Build history of the part. All positions in model axes, mm. Give positions to 0.01 mm unless a question says otherwise; leave off trailing zeros. Loops run counter-clockwise (first coordinate to the right, second up) from the corner with the lowest first, then second, coordinate; pieces in that order, holes last. Notation, with made-up numbers: (75.5, 34.25) -> (99.5, 34.25) arc R30 cw to (99.5, 56.25) -> close; hole circle Ø7 at (-21.75, 68). An arc over 180 degrees is marked (long way). Answer as a JSON object with one key per item and string values. Group by question number.
Q1. Wall check: probe 1 along X at (y, z) = (4.75, -79); probe 2 along Z at (x, y) = (76.5, 4.75); probe 3 along X at (y, z) = (4, -57.5). Give the ranges that are in metal, low to high. Write a range as from..to.
Q2. Band-saw the part on C-C, the plane z = -70. Write the cut outline in (x, y).
Q3. Drop a flat-ended pin along its axis: pin 1 (3.5 mm diameter, centred on x = 33.35, z = -32.5, fed in from +Y). Give the stop position or say it passes through.
Q4. Band-saw the part on D-D, the plane y = 5.25. Count the separate pieces of the cut face and the enclosed holes in it, plus the area to 3 significant figures.
Q5. Two-plate mould, pull along Z, no slides. Class faces 1 (the cylindrical face through (88.67, 3.22, -78.67)), 2 (the cylindrical face through (75, 3.2, -34.7)), 3 (the flat face through (54, 3, -90)), 4 (the flat face through (54, 0, -46)): pulls with the +Z half, pulls with the -Z half, needs draft (parallel to the pull), parting line crosses it, or undercut.
Q6. Band-saw the part on B-B, the plane z = -57.5. Write the cut outline in (x, y).
Q7. Band-saw the part on A-A, the plane x = 55. Write the cut outline in (y, z).
from build123d import *

# Parameters (mm, degrees)
SKETCH2_W            = 110
SKETCH2_H            = 90
BOSS_EXTRUDE1_DEPTH  = 6.35
SKETCH3_R            = 2.5
MOUNTING_HOLES_DEPTH = 143.268487375
SKETCH4_R            = 2.75
CUT_EXTRUDE1_DEPTH   = 143.268487375


with BuildPart() as part:
    # Sketch2 → Boss-Extrude1 (new body)
    with BuildSketch(Plane(origin=(0, 0, 0), x_dir=(1, 0, 0), z_dir=(0, 1, 0))):
        with Locations((55, 45)):
            Rectangle(SKETCH2_W, SKETCH2_H)
    extrude(amount=BOSS_EXTRUDE1_DEPTH)

    # Sketch3 → Mounting Holes (cut, through all)
    with BuildSketch(Plane(origin=(0, 6.35, 0), x_dir=(1, 0, 0), z_dir=(0, 1, 0))):
        with Locations(Location((18.85, 79, 0), (0, 0, 270))):
            Circle(SKETCH3_R)
        with Locations(Location((18.85, 11, 0), (0, 0, 90))):
            Circle(SKETCH3_R)
        with Locations(Location((91.15, 11, 0), (0, 0, 270))):
            Circle(SKETCH3_R)
        with Locations(Location((91.15, 79, 0), (0, 0, 90))):
            Circle(SKETCH3_R)
    extrude(amount=-MOUNTING_HOLES_DEPTH, mode=Mode.SUBTRACT)

    # Sketch4 → Cut-Extrude1 (cut, through all)
    with BuildSketch(Plane(origin=(0, 6.35, 0), x_dir=(1, 0, 0), z_dir=(0, 1, 0))):
        with Locations(Location((55, 70, 0), (0, 0, 270))):
            Circle(SKETCH4_R)
        with Locations(Location((76.650635095, 57.5, 0), (0, 0, 270))):
            Circle(SKETCH4_R)
        with Locations(Location((76.650635095, 32.5, 0), (0, 0, 270))):
            Circle(SKETCH4_R)
        with Locations(Location((55, 20, 0), (0, 0, 270))):
            Circle(SKETCH4_R)
        with Locations(Location((33.349364905, 32.5, 0), (0, 0, 270))):
            Circle(SKETCH4_R)
        with Locations(Location((33.349364905, 57.5, 0), (0, 0, 270))):
            Circle(SKETCH4_R)
    extrude(amount=-CUT_EXTRUDE1_DEPTH, mode=Mode.SUBTRACT)


solid = part.part
Worked answers:
{
 "1": {"probe 1": "0..16.35, 21.35..88.65, 93.65..110", "probe 2": "-90..-60.25, -54.75..-35.25, -29.75..0", "probe 3": "0..30.6, 36.1..73.9, 79.4..110"},
 "2": {"outline": "(0, 0) -> (52.25, 0) -> (52.25, 6.35) -> (0, 6.35) -> close; (57.75, 0) -> (110, 0) -> (110, 6.35) -> (57.75, 6.35) -> close"},
 "3": {"pin 1": "through"},
 "4": {"separate pieces": "1", "enclosed holes": "10", "area": "9,680 mm2"},
 "5": {"face 1": "undercut", "face 2": "undercut", "face 3": "pulls with the -Z half", "face 4": "needs draft"},
 "6": {"outline": "(0, 0) -> (30.6, 0) -> (30.6, 6.35) -> (0, 6.35) -> close; (36.1, 0) -> (73.9, 0) -> (73.9, 6.35) -> (36.1, 6.35) -> close; (79.4, 0) -> (110, 0) -> (110, 6.35) -> (79.4, 6.35) -> close"},
 "7": {"outline": "(0, -90) -> (6.35, -90) -> (6.35, -72.75) -> (0, -72.75) -> close; (0, -67.25) -> (6.35, -67.25) -> (6.35, -22.75) -> (0, -22.75) -> close; (0, -17.25) -> (6.35, -17.25) -> (6.35, 0) -> (0, 0) -> close"}
}
